Can you work these out from the model? Positions are in its coordinate system, mm. A direction names the side the tool comes from. Round coordinates to 2 decimals unless told otherwise and drop trailing zeros. Loops run counter-clockwise (first coordinate to the right, second up) from the corner with the lowest first, then second, coordinate; pieces in that order, holes last. Notation, with made-up numbers: (66, 84.25) -> (90, 84.25) arc R23 ccw to (90, 96.25) -> close; hole circle Ø11 at (-16, 10). An arc over 180 degrees is marked (long way). Answer as a JSON object with one key per item and string values.
Autodesk Inventor part; units mm, degrees
ref_plane "YZ Plane" through (0, 0, 0) normal (1, 0, 0) x (0, 1, 0)
ref_plane "XZ Plane" through (0, 0, 0) normal (0, 1, 0) x (-1, 0, 0)
ref_plane "XY Plane" through (0, 0, 0) normal (0, 0, 1) x (1, 0, 0)
sketch "スケッチ1" plane through (0, 0, 0) normal (0, 1, 0) x (-1, 0, 0)
  line L0 (-29, -17.95) -> (29, -17.95)
  line L1 (29, -17.95) -> (29, 17.95)
  line L2 (29, 17.95) -> (-29, 17.95)
  line L3 (-29, 17.95) -> (-29, -17.95)
  line L4 (-29, -17.95) -> (29, 17.95) construction
  line L5 (29, -17.95) -> (-29, 17.95) construction
  point P0 (0, 0)
  dimension "d0" = 35.9
  dimension "d1" = 58
extrude "プレート1" add sketch "スケッチ1" along normal blind 2
sketch "スケッチ2" plane through (29, 0, 17.95) normal (1, 0, 0) x (0, 0, -1)
  line L0 (0, 2) -> (35.9, 2)
  line L1 (35.9, 2) -> (0, 2)
  line L2 (0, 2) -> (0, 32)
  line L3 (0, 32) -> (35.9, 32)
  line L4 (35.9, 32) -> (35.9, 2)
  point P0 (17.95, 0)
  dimension "d3" = 30
sheet face with bend "面2" sketch "スケッチ2" thickness 2 toward (1, 0, 0) bend radius 2
bend "曲げ1"
sketch "スケッチ3" plane through (-29, 0, -17.95) normal (-1, 0, 0) x (0, 0, 1)
  line L0 (0, 0) -> (0, 2)
  line L1 (0, 32) -> (35.9, 32)
  line L2 (0, 2) -> (35.9, 2)
  line L3 (35.9, 2) -> (35.9, 32)
  line L4 (35.9, 32) -> (0, 32)
  line L5 (0, 32) -> (0, 2)
  point P0 (17.95, 0)
sheet face with bend "面3" sketch "スケッチ3" thickness 2 toward (-1, 0, 0) bend radius 2
bend "曲げ2"
sketch "スケッチ4" plane through (-31, 0, -17.95) normal (-1, 0, 0) x (0, 0, 1)
  line L0 (6, 28) -> (6, 8)
  arc A0 (6, 8) -> (10, 8) centre (8, 8) ccw
  line L1 (10, 8) -> (10, 28)
  arc A1 (10, 28) -> (6, 28) centre (8, 28) ccw
  line L2 (0, 32) -> (35.9, 32)
  line L3 (35.9, 4) -> (0, 4)
  line L4 (0, 4) -> (0, 32)
  line L5 (25.9, 28) -> (25.9, 8)
  arc A2 (25.9, 8) -> (29.9, 8) centre (27.9, 8) ccw
  line L6 (29.9, 8) -> (29.9, 28)
  arc A3 (29.9, 28) -> (25.9, 28) centre (27.9, 28) ccw
  line L7 (35.9, 32) -> (35.9, 4)
  point P0 (17.95, 0)
  dimension "d14" = 2
  dimension "d15" = 4
  dimension "d16" = 4
  dimension "d17" = 6
  dimension "d18" = 2
  dimension "d19" = 6
extrude "押し出し1" cut sketch "スケッチ4" against normal blind 100 contours A1 L1 A0 L0 | A3 L6 A2 L5
sketch "スケッチ5" plane through (0, 2, 0) normal (0, 1, 0) x (1, 0, 0)
  line L0 (-21, -9.95) -> (21, -9.95)
  arc A0 (21, -9.95) -> (21, -5.95) centre (21, -7.95) ccw
  line L1 (21, -5.95) -> (-21, -5.95)
  arc A1 (-21, -5.95) -> (-21, -9.95) centre (-21, -7.95) ccw
  line L2 (-21, 5.95) -> (21, 5.95)
  arc A2 (21, 5.95) -> (21, 9.95) centre (21, 7.95) ccw
  line L3 (21, 9.95) -> (-21, 9.95)
  arc A3 (-21, 9.95) -> (-21, 5.95) centre (-21, 7.95) ccw
  line L4 (-27, 17.95) -> (27, 17.95)
  line L5 (27, -17.95) -> (-27, -17.95)
  line L6 (-27, 17.95) -> (-27, -17.95)
  line L7 (27, -17.95) -> (27, 17.95)
  point P0 (0, 0)
  dimension "d22" = 2
  dimension "d23" = 2
  dimension "d25" = 10
  dimension "d26" = 10
  dimension "d27" = 6
  dimension "d28" = 6
  dimension "d29" = 6
  dimension "d30" = 6
extrude "押し出し2" cut sketch "スケッチ5" against normal blind 3 contours A1 L1 A0 L0 | A3 L3 A2 L2
equation "\"d2\" = Thickness"
equation "\"d4\" = BendRadius"
equation "\"d5\" = BendReliefWidth"
equation "\"d7\" = MinimumRemnant"
equation "\"d6\" = BendReliefDepth"
equation "\"d8\" = TransitionRadius"
equation "\"d9\" = BendRadius"
equation "\"d10\" = BendReliefWidth"
equation "\"d12\" = MinimumRemnant"
equation "\"d11\" = BendReliefDepth"
equation "\"d13\" = TransitionRadius"
equation "\"BendRadius\" = Thickness"
equation "\"BendReliefWidth\" = Thickness"
equation "\"BendReliefDepth\" = 0.5 * Thickness"
equation "\"CornerReliefSize\" = 4 * Thickness"
equation "\"MinimumRemnant\" = 2 * Thickness"
equation "\"TransitionRadius\" = BendRadius"
equation "\"JacobiRadiusSize\" = BendRadius"
equation "\"GapSize\" = Thickness"
properties part number "trackball_cup" material "アルミニウム 6061"
Q1. I want a section at C-C, the plane x = 26. Write out the boundary of the cut face in (y, z).
Determined:
{"outline": "(0, -17.95) -> (2, -17.95) -> (2, 17.95) -> (0, 17.95) -> close"}
Q2. We'd pull the mould along Z, two halves only. Please class faces 1 (the flat face through (29, 18, 0)), 2 (the flat face through (-30, 18, -11.95)): pulls with the +Z half, pulls with the -Z half, needs draft (parallel to the pull), parting line crosses it, or undercut.
Determined:
{"face 1": "needs draft", "face 2": "undercut"}
Q3. If I drill on L1, parallel to X at y = 6.5, z = -1; L2, parallel to Y at x = -4.5, z = 1.5; L3, parallel to X at y = 3, z = 14, over which ranges is the centre line in solid material (lowest first)? Write a range as [from, to].
Determined:
{"L1": "[-31, -29], [29, 31]", "L2": "[0, 2]", "L3": "[-30.87, -28.73], [28.73, 30.87]"}
Q4. On a 3-axis mill with a long thin cutter (end or side, diameter ignored), from which of +Z, -Z, +X, -X, +Y, -Y can I reach the whole of each face in a straight line? I mean faces 3 (the flat face through (-30, 32, 0)), 4 (the cylindrical face through (23, 1, -8)), 5 (the flat face through (-29, 18, 0)), 6 (the flat face through (31, 18, 0)), 7 (the flat face through (30, 18, -11.95)). Say none if no direction works.
Determined:
{"face 3": "+Z, -Z, +X, -X, +Y", "face 4": "+Y, -Y", "face 5": "+Z, -Z, +Y", "face 6": "+Z, -Z, +X, +Y, -Y", "face 7": "+X, -X"}
Q5. I want a section at B-B, the plane z = 15. Write out the boundary of the cut face in (x, y), then the cut area to 3 significant figures.
Determined:
{"outline": "(-31, 4) arc R4 ccw to (-27, 0) -> (27, 0) arc R4 ccw to (31, 4) -> (31, 32) -> (29, 32) -> (29, 4) arc R2 cw to (27, 2) -> (-27, 2) arc R2 cw to (-29, 4) -> (-29, 32) -> (-31, 32) -> close", "area": "239 mm²"}
Q6. I'm going to push flat-ended pins straight in: pin 1 (18 mm diameter, centred on x = -7.5, z = -5.5, fed in from +Y); pin 2 (10 mm diameter, centred on x = 20.5, y = 24, fed in from +Z). Where does each tip first touch, or does it pass through?
Determined:
{"pin 1": "y = 2", "pin 2": "through"}
Q7. I want a section at A-A, the plane y = 12.5. Write out the boundary of the cut face in (x, z).
Determined:
{"outline": "(-31, -17.95) -> (-29, -17.95) -> (-29, -11.95) -> (-31, -11.95) -> close; (-31, -7.95) -> (-29, -7.95) -> (-29, 7.95) -> (-31, 7.95) -> close; (-31, 11.95) -> (-29, 11.95) -> (-29, 17.95) -> (-31, 17.95) -> close; (29, -17.95) -> (31, -17.95) -> (31, -11.95) -> (29, -11.95) -> close; (29, -7.95) -> (31, -7.95) -> (31, 7.95) -> (29, 7.95) -> close; (29, 11.95) -> (31, 11.95) -> (31, 17.95) -> (29, 17.95) -> close"}
